Geometry check sheet. Reference: the model listing, model coordinates, mm. Face numbers are marked on the shaded views. A direction names the side the tool comes from. Give positions to 0.01 mm unless a question says otherwise; leave off trailing zeros. Write each loop counter-clockwise with the first axis right and the second up, starting at its lowest first coordinate (ties: lowest second). Pieces come first, ordered by that corner, then holes.
(1) Cross-section at B-B (z = -6). Record the boundary of the cut face in (x, y).
(2) Tool access check on the marked faces 1 and 2. Record the directions out of +Z, -Z, +X, -X, +Y, -Y that give a thin tool (end or side, any length) a straight path to the whole face; none if there is none.
(3) Cross-section at A-A (y = 6.5). Record the boundary of the cut face in (x, z), and give its area (3 significant figures).
(4) Depth check by flat-ended pin: P1, Ø8, axis at y = -4, z = 1.5, coming from the -X side; P2, Ø10, axis at x = 30, y = 6, coming from the -Z side; P3, Ø1, axis at y = 6.5, z = -2, coming from the -X side. Enter the tip coordinate at first touch or a pass-through.
(5) Thickness scan on line 1 along Z through (x, y) = (143.75, 0); line 2 along Y through (x, z) = (16.5, 6). Record the ranges inside material, lowest first.
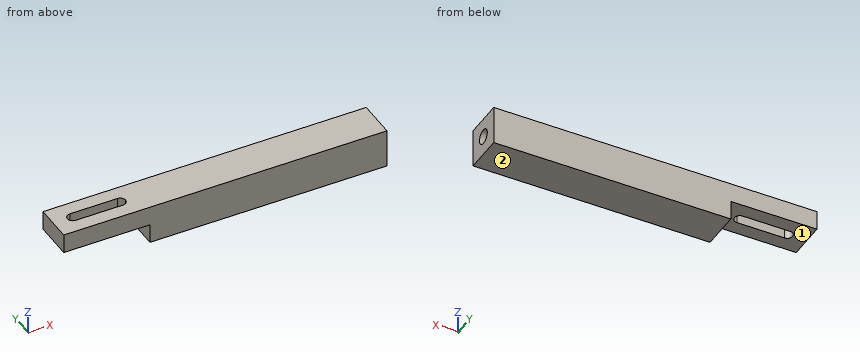
```python
from build123d import *

# Parameters (mm, degrees)
F0_W     = 18
F0_H     = 18
F1_DEPTH = 150
F2_W     = 40
F2_H     = 18
F3_DEPTH = 9
F4_DEPTH = 25
F6_D     = 6.8
F6_DEPTH = 18.75
F6_TIP   = 2.0429261047


with BuildPart() as f1:
    # F0 (on Right) → F1 (new body)
    with BuildSketch(Plane.YZ):
        Rectangle(F0_W, F0_H)
    extrude(amount=F1_DEPTH)

    # F2 (on face) → F3 (cut)
    with BuildSketch(Plane(origin=(0, 0, -9), x_dir=(1, 0, 0), z_dir=(0, 0, -1))):
        with Locations((20, 0)):
            Rectangle(F2_W, F2_H)
        with BuildLine():
            ThreePointArc((9, -2.5), (6.5, 0), (9, 2.5))
            Line((9, 2.5), (31, 2.5))
            ThreePointArc((31, 2.5), (32.767766953, 1.767766953), (33.5, 0))
            ThreePointArc((33.5, 0), (32.767766953, -1.767766953), (31, -2.5))
            Line((31, -2.5), (9, -2.5))
        make_face(mode=Mode.SUBTRACT)
    extrude(amount=-F3_DEPTH, mode=Mode.SUBTRACT)

    # F4 (cut): a face of the model
    f4_faces = [f1.faces().sort_by_distance(p)[0] for p in [
        (20, 0, -9),
    ]]
    extrude(f4_faces, amount=-F4_DEPTH, mode=Mode.SUBTRACT)

    # F6
    with Locations(Plane.YZ.offset(150)):
        with Locations((0, 0)):
            Hole(F6_D / 2, depth=F6_DEPTH)
            with Locations((0, 0, -(F6_DEPTH + F6_TIP / 2))):  # 118° drill point
                Cone(0, F6_D / 2, F6_TIP, mode=Mode.SUBTRACT)


solid = f1.part
```
Reply:
1. outline: (40, -9) - (150, -9) - (150, 9) - (40, 9) - close
2. face 1: -Z, -X, +Y, -Y
2. face 2: -Z, +X, -X, +Y, -Y
3. outline: (0, 0) - (40, 0) - (40, -9) - (150, -9) - (150, 9) - (0, 9) - close
3. area: 2,340 mm2
4. P1: stops at x = 0
4. P2: stops at z = 0
4. P3: stops at x = 40
5. line 1: z = -9 to -3.4, 3.4 to 9
5. line 2: y = -9 to -2.5, 2.5 to 9
